Can you work these out from the model? Positions are in its coordinate system, mm. Face numbers are marked on the shaded views. A direction names the side the tool comes from. Round coordinates to 2 decimals unless told otherwise and drop trailing zeros. Write each loop counter-clockwise with the first axis right and the second up, starting at its lowest first coordinate (ties: lowest second). Pieces come first, ordered by that corner, then holes. Notation, with made-up numbers: (-1.75, -0.5) -> (56.25, -0.5) arc R23 ccw to (56.25, 29.5) -> close; hole circle Ø2 at (34.25, 1). An arc over 180 degrees is marked (long way). Write item = value, one per line. Start each with the question number.
1) Imagine slicing it at B-B, the plane x = 0. Please give me the cut outline in (y, z).
2) If I drill on line 1 (X direction, y = 13.25, z = 0); line 2 (Y direction, x = 4, z = -1.75); line 3 (Z direction, x = 0, y = 12.75), over which ranges is the centre line in solid material (lowest first)?
3) I'm going to push flat-ended pins straight in: pin 1 (3 mm diameter, centred on y = 15.45, z = 0.05, fed in from +X); pin 2 (1.5 mm diameter, centred on y = 15, z = -4.5, fed in from +X). Where does each tip first touch, or does it pass through?
4) Imagine slicing it at D-D, the plane z = 3. Please give me the cut outline in (x, y).
5) Thinking about a two-plate mould opening in Y: for the marked faces 1, 2 and 3, which applies, +Y half, -Y half, draft (parallel to the pull), parting line (faces both ways), or undercut?
6) For the marked faces 4, 5 and 6, which set-ups out of +Z, -Z, +X, -X, +Y, -Y let a thin tool reach every point of the face, with its end or its side?
7) Imagine slicing it at A-A, the plane z = 1.5. Please give me the cut outline in (x, y).
8) Imagine slicing it at C-C, the plane x = 4. Please give me the cut outline in (y, z), then the cut area to 3 significant figures.
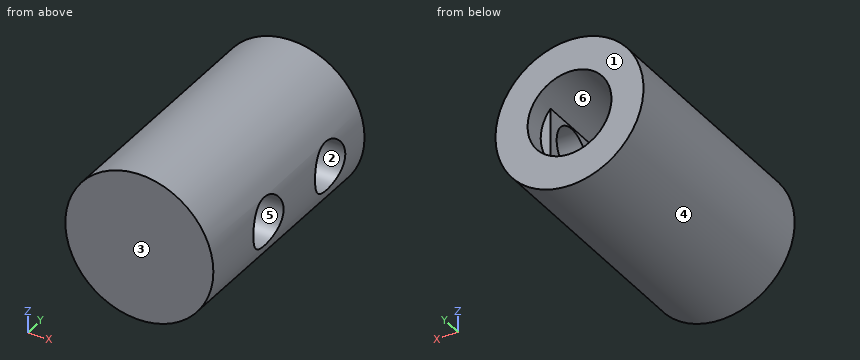
from build123d import *

# Parameters (mm, degrees)
SKETCH1_R           = 6
BOSS_EXTRUDE1_DEPTH = 20
SKETCH2_R           = 3.4
CUT_EXTRUDE1_DEPTH  = 13.55
SKETCH5_W           = 1.550685087
SKETCH5_H           = 7.184215806
BOSS_EXTRUDE2_DEPTH = 13.55
SKETCH6_R           = 2
CUT_EXTRUDE2_DEPTH  = 13.55


with BuildPart() as part:
    # Sketch1 → Boss-Extrude1 (new body)
    with BuildSketch(Plane(origin=(0, 0, 0), x_dir=(1, 0, 0), z_dir=(0, 1, 0))):
        Circle(SKETCH1_R)
    extrude(amount=BOSS_EXTRUDE1_DEPTH)

    # Sketch2 → Cut-Extrude1 (cut)
    with BuildSketch(Plane(origin=(0, 20, 0), x_dir=(1, 0, 0), z_dir=(0, 1, 0))):
        Circle(SKETCH2_R)
    extrude(amount=-CUT_EXTRUDE1_DEPTH, mode=Mode.SUBTRACT)

    # Sketch5 → Boss-Extrude2 (add)
    with BuildSketch(Plane(origin=(0, 18.26, 0), x_dir=(1, 0, 0), z_dir=(0, 1, 0))):
        with Locations((3.375342544, 0.020519704)):
            Rectangle(SKETCH5_W, SKETCH5_H)
    extrude(amount=-BOSS_EXTRUDE2_DEPTH)

    # Sketch6 → Cut-Extrude2 (cut)
    with BuildSketch(Plane.ZY.offset(-2.6)):
        with Locations((0.054169736, 15.452187313)):
            Circle(SKETCH6_R)
        with Locations((0, 7.29207964)):
            Circle(SKETCH6_R)
    extrude(amount=-CUT_EXTRUDE2_DEPTH, mode=Mode.SUBTRACT)


solid = part.part
Reported:
q1.outline = (0, -6) -> (20, -6) -> (20, -3.4) -> (6.45, -3.4) -> (6.45, 3.4) -> (20, 3.4) -> (20, 6) -> (0, 6) -> close
q2.line_1 = -6 to -3.4, 2.6 to 6
q2.line_2 = 0 to 6.32, 8.26 to 14.59, 16.32 to 20
q2.line_3 = -6 to -3.4, 3.4 to 6
q3.pin_1 = -3.03
q3.pin_2 = 4.68
q4.outline = (-5.2, 0) -> (5.2, 0) -> (5.2, 20) -> (1.6, 20) -> (1.6, 6.45) -> (-1.6, 6.45) -> (-1.6, 20) -> (-5.2, 20) -> close
q5.face_1 = +Y half
q5.face_2 = undercut
q5.face_3 = -Y half
q6.face_4 = +Y, -Y
q6.face_5 = +X
q6.face_6 = +Y
q7.outline = (-5.81, 0) -> (5.81, 0) -> (5.81, 5.97) -> (2.6, 5.97) -> (2.6, 6.45) -> (-3.05, 6.45) -> (-3.05, 20) -> (-5.81, 20) -> close; (2.6, 8.61) -> (5.81, 8.61) -> (5.81, 14.07) -> (2.6, 14.07) -> close; (2.6, 16.83) -> (5.81, 16.83) -> (5.81, 20) -> (3.05, 20) -> (3.05, 18.26) -> (2.6, 18.26) -> close
q8.outline = (0, -4.47) -> (20, -4.47) -> (20, 4.47) -> (0, 4.47) -> close; hole circle Ø4 at (7.29, 0); hole circle Ø4 at (15.45, 0.05)
q8.area = 154 mm²
